The listing builds one solid part. Answer for the finished solid, in the listing's coordinates (mm). A direction names the side the tool comes from. Coordinates: 2 decimals unless noted, no trailing zeros. Order: outer loops, then holes, each group sorted by start corner. A loop starts at its lowest first (then second) coordinate and runs counter-clockwise, first axis right, second up. Notation, with made-up numbers: (68, 50) - (73, 50) arc R18 ccw to (73, 67) - close; hole circle Ø5 at (4.5, -36). An arc over 180 degrees is marked (long way). Use a Markdown table: item, result. Add a question column.
Item 1: The mould has two halves that part along Z. Classify faces 1 (the flat face through (-11, 24, 20.75)), 2 (the flat face through (-17, 18, -20.75)), 3 (the cylindrical face through (2.526, 0.53, -1.667)): released by +Z, released by -Z, zero draft, split by the parting line, or undercut.
Item 2: For faces 4 (the flat face through (-16, 2, 24)), 5 (the flat face through (-16, 2, -24)), 6 (the flat face through (12, 13, -20.75)), 7 (the cylindrical face through (4.66, 2.14, -3.6)), 8 (the flat face through (10.35, 15, -24)), determine the directions among +Z, -Z, +X, -X, +Y, -Y from which every point of the face is accessible in a straight line to the end or side of a thin tool.
Item 3: The part is cut by section A-A, the plane z = -24.8. Give the vertices of the cut face in (x, y) (3 decimals), then the cut area to 3 significant figures.
Item 4: The part is cut by section C-C, the plane y = 13.43. Give the vertices of the cut face in (x, z).
Item 5: The part is cut by section B-B, the plane x = 3.6. Give the vertices of the cut face in (y, z) (3 decimals), then the cut area to 3 significant figures.
Item 6: The part is cut by section D-D, the plane z = 17. Give the vertices of the cut face in (x, y) (3 decimals), then the cut area to 3 significant figures.
Item 7: Flat-ended cylindrical pins translate along their axes: P1, Ø3.5, axis at y = 2.5, z = 24, coming from the -X side; P2, Ø10.5, axis at y = 16, z = -3, coming from the +X side; P3, Ø3.5, axis at x = 3.6, z = 1.91, coming from the +Y side (3 decimals). Find the tip coordinate at first contact, or state that the pin passes through.
Item 8: Find the intervals of material crossed by line 1 along Y through (x, z) = (-13.5, 1) (3 decimals); line 2 along Z through (x, y) = (3.6, 2.65); line 3 along Y through (x, z) = (18.5, 25) (3 decimals), in increasing order.
from build123d import *

# Parameters (mm, degrees)
SKETCH1_W           = 40
SKETCH1_H           = 55.6
BOSS_EXTRUDE1_DEPTH = 3.175
SKETCH2_W           = 4
SKETCH2_H           = 41.5
SKETCH2_H_2         = 7.05
BOSS_EXTRUDE2_DEPTH = 20.6
BOSS_EXTRUDE3_DEPTH = 3.175
SKETCH5_R           = 2.25
CUT_EXTRUDE2_DEPTH  = 4
SKETCH6_R           = 1.65
CUT_EXTRUDE3_DEPTH  = 4
FILLET1_R           = 1
SKETCH7_W           = 4
SKETCH7_H           = 7.05
CUT_EXTRUDE4_DEPTH  = 3.175
FILLET2_R           = 1
SKETCH8_R           = 1.1
CUT_EXTRUDE6_DEPTH  = 3.175
CUT_EXTRUDE7_DEPTH  = 2.1
CUT_EXTRUDE8_START  = 23.775
CUT_EXTRUDE8_DEPTH  = 23.775


with BuildPart() as part:
    # Sketch1 → Boss-Extrude1 (new body)
    with BuildSketch(Plane(origin=(0, 0, 0), x_dir=(1, 0, 0), z_dir=(0, 1, 0))):
        Rectangle(SKETCH1_W, SKETCH1_H)
    extrude(amount=BOSS_EXTRUDE1_DEPTH)

    # Sketch2 → Boss-Extrude2 (add)
    with BuildSketch(Plane(origin=(0, 3.175, 0), x_dir=(1, 0, 0), z_dir=(0, 1, 0))):
        with Locations((-18, 0)):
            Rectangle(SKETCH2_W, SKETCH2_H)
        with Locations((12.35, 24.275)):
            Rectangle(SKETCH2_W, SKETCH2_H_2)
        with Locations((12.35, -24.275)):
            Rectangle(SKETCH2_W, SKETCH2_H_2)
    extrude(amount=BOSS_EXTRUDE2_DEPTH)

    # Sketch3 → Boss-Extrude3 (add)
    with BuildSketch(Plane(origin=(0, 23.775, 0), x_dir=(1, 0, 0), z_dir=(0, 1, 0))):
        Polygon((-20, 20.75), (10.35, 20.75), (10.35, 27.8), (14.35, 27.8), (14.35, -27.8), (10.35, -27.8), (10.35, -20.75), (-20, -20.75), align=None)
    extrude(amount=BOSS_EXTRUDE3_DEPTH)

    # Sketch5 → Cut-Extrude2 (cut)
    with BuildSketch(Plane(origin=(14.35, 0, 0), x_dir=(0, 0, -1), z_dir=(1, 0, 0))):
        with Locations((-24.8, 8.425)):
            Circle(SKETCH5_R)
        with Locations((-24.8, 18.425)):
            Circle(SKETCH5_R)
        with Locations((24.8, 18.425)):
            Circle(SKETCH5_R)
        with Locations((24.8, 8.425)):
            Circle(SKETCH5_R)
    extrude(amount=-CUT_EXTRUDE2_DEPTH, mode=Mode.SUBTRACT)

    # Sketch6 → Cut-Extrude3 (cut)
    with BuildSketch(Plane.ZY.offset(20)):
        with Locations((10, 13.43)):
            Circle(SKETCH6_R)
    extrude(amount=-CUT_EXTRUDE3_DEPTH, mode=Mode.SUBTRACT)

    # Fillet1
    fillet1_edges = [part.edges().sort_by_distance(p)[0] for p in [
        (14.35, 13.475, 20.75),
        (14.35, 13.475, -20.75),
    ]]
    fillet(fillet1_edges, radius=FILLET1_R)

    # Sketch7 → Cut-Extrude4 (cut)
    with BuildSketch(Plane(origin=(0, 3.175, 0), x_dir=(1, 0, 0), z_dir=(0, 1, 0))):
        with Locations((-18, -24.275)):
            Rectangle(SKETCH7_W, SKETCH7_H)
        with Locations((-18, 24.275)):
            Rectangle(SKETCH7_W, SKETCH7_H)
    extrude(amount=-CUT_EXTRUDE4_DEPTH, mode=Mode.SUBTRACT)

    # Fillet2
    fillet2_edges = [part.edges().sort_by_distance(p)[0] for p in [
        (-16, 1.5875, 20.75),
        (-16, 1.5875, 27.8),
        (-16, 1.5875, -27.8),
        (-16, 1.5875, -20.75),
    ]]
    fillet(fillet2_edges, radius=FILLET2_R)

    # Sketch8 → Cut-Extrude6 (cut)
    with BuildSketch(Plane.XZ):
        with Locations(Location((3.6, 1.905255888, 0), (0, 0, 270))):
            Circle(SKETCH8_R)
        with Locations(Location((3.6, -1.905255888, 0), (0, 0, 270))):
            Circle(SKETCH8_R)
        with Locations(Location((0.3, 0, 0), (0, 0, 270))):
            Circle(SKETCH8_R)
    extrude(amount=-CUT_EXTRUDE6_DEPTH, mode=Mode.SUBTRACT)

    # Sketch9 → Cut-Extrude7 (cut)
    with BuildSketch(Plane(origin=(0, 3.175, 0), x_dir=(1, 0, 0), z_dir=(0, 1, 0))):
        with BuildLine():
            ThreePointArc((1.645861873, -1.479410632), (4.6, -3.637306696), (4.208276253, 0))
            ThreePointArc((4.208276253, 0), (4.6, 3.637306696), (1.645861873, 1.479410632))
            ThreePointArc((1.645861873, 1.479410632), (-1.7, 0), (1.645861873, -1.479410632))
        make_face()
    extrude(amount=-CUT_EXTRUDE7_DEPTH, mode=Mode.SUBTRACT)

    # Sketch10 → Cut-Extrude8 (cut)
    with BuildSketch(Plane(origin=(0, 3.175, 0), x_dir=(1, 0, 0), z_dir=(0, 1, 0)).offset(CUT_EXTRUDE8_START)):
        with BuildLine():
            ThreePointArc((1.645861873, -1.479410632), (4.6, -3.637306696), (4.208276253, 0))
            ThreePointArc((4.208276253, 0), (4.6, 3.637306696), (1.645861873, 1.479410632))
            ThreePointArc((1.645861873, 1.479410632), (-1.7, 0), (1.645861873, -1.479410632))
        make_face()
    extrude(amount=-CUT_EXTRUDE8_DEPTH, mode=Mode.SUBTRACT)


solid = part.part
Solution:
| question | item | result |
|---|---|---|
| 1 | face 1 | released by +Z |
| 1 | face 2 | released by -Z |
| 1 | face 3 | undercut |
| 2 | face 4 | +Z, -X, +Y, -Y |
| 2 | face 5 | -Z, -X, +Y, -Y |
| 2 | face 6 | +X |
| 2 | face 7 | +Y |
| 2 | face 8 | -Z, -X, +Y |
| 3 | outline | (-16, 0) - (20, 0) - (20, 3.175) - (14.35, 3.175) - (14.35, 6.175) - (10.35, 6.175) - (10.35, 3.175) - (-16, 3.175) - close; (10.35, 10.675) - (14.35, 10.675) - (14.35, 16.175) - (10.35, 16.175) - close; (10.35, 20.675) - (14.35, 20.675) - (14.35, 26.95) - (10.35, 26.95) - close |
| 3 | area | 173 mm2 |
| 4 | outline | (-20, -20.75) - (-16, -20.75) - (-16, 8.35) - (-20, 8.35) - close; (-20, 11.65) - (-16, 11.65) - (-16, 20.75) - (-20, 20.75) - close; (10.35, -27.8) - (14.35, -27.8) - (14.35, -21.75) arc R1 ccw to (13.35, -20.75) - (10.35, -20.75) - close; (10.35, 20.75) - (13.35, 20.75) arc R1 ccw to (14.35, 21.75) - (14.35, 27.8) - (10.35, 27.8) - close |
| 5 | outline | (0, -27.8) - (3.175, -27.8) - (3.175, -3.905) - (1.075, -3.905) - (1.075, -3.005) - (0, -3.005) - close; (0, -0.805) - (1.075, -0.805) - (1.075, 0.805) - (0, 0.805) - close; (0, 3.005) - (1.075, 3.005) - (1.075, 3.905) - (3.175, 3.905) - (3.175, 27.8) - (0, 27.8) - close; (23.775, -20.75) - (26.95, -20.75) - (26.95, -3.905) - (23.775, -3.905) - close; (23.775, 3.905) - (26.95, 3.905) - (26.95, 20.75) - (23.775, 20.75) - close |
| 5 | area | 262 mm2 |
| 6 | outline | (-20, 0) - (20, 0) - (20, 3.175) - (-16, 3.175) - (-16, 23.775) - (14.35, 23.775) - (14.35, 26.95) - (-20, 26.95) - close |
| 6 | area | 318 mm2 |
| 7 | P1 | stops at x = -16 |
| 7 | P2 | stops at x = -16 |
| 7 | P3 | stops at y = 1.075 |
| 8 | line 1 | y = 0 to 3.175, 23.775 to 26.95 |
| 8 | line 2 | z = -27.8 to -3.91, 3.91 to 27.8 |
| 8 | line 3 | y = 0 to 3.175 |
